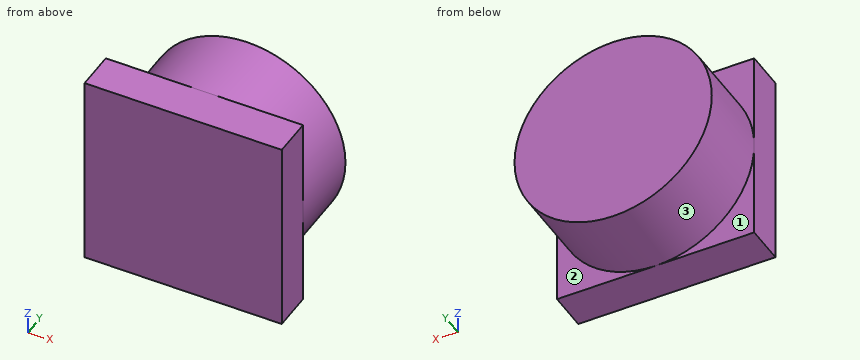
Autodesk Inventor part; units mm, degrees
ref_plane "YZ Plane" through (0, 0, 0) normal (1, 0, 0) x (0, 1, 0)
ref_plane "XZ Plane" through (0, 0, 0) normal (0, 1, 0) x (-1, 0, 0)
ref_plane "XY Plane" through (0, 0, 0) normal (0, 0, 1) x (1, 0, 0)
sketch "Skizze1" plane through (0, 0, 0) normal (0, 1, 0) x (-1, 0, 0)
  circle A0 centre (0, 0) radius 25
  dimension "d0" = 50
extrude "Extrusion1" add sketch "Skizze1" along normal blind 20
sketch "Skizze2" plane through (0, 0, 0) normal (0, -1, 0) x (1, 0, 0)
  line L0 (-25, 25) -> (25, 25)
  line L1 (25, 25) -> (25, -25)
  line L2 (25, -25) -> (-25, -25)
  line L3 (-25, -25) -> (-25, 25)
  circle A0 centre (0, 0) radius 25
extrude "Extrusion2" add sketch "Skizze2" along normal blind 10
equation "\"d0\" = UsedParameter"
equation "\"UsedParameter\" = 50"
equation "\"unusedParameter\" = 1"
properties part number "2Extrusionen"
Read the model definition and answer for the solid it produces. Units are mm, in the model's axes. Face numbers are marked on the shaded views. A direction names the side the tool comes from. Give positions to 0.01 mm unless a question says otherwise; leave off trailing zeros. Write each loop counter-clockwise with the first axis right and the second up, starting at its lowest first coordinate (ties: lowest second). Pieces come first, ordered by that corner, then holes. Notation, with made-up numbers: M 60,-25 L 82,-25 A33 cw 82,3 Z; hole C 42,4 d6. An arc over 180 degrees is marked long. Put each result on its own line as item: value. Start each with the question number.
1. The part is cut by section A-A, the plane x = 10.5. Give the vertices of the cut face in (y, z).
2. The part is cut by section B-B, the plane y = 8.25. Give the vertices of the cut face in (x, z).
3. Each of these flat-tipped pins is pushed along its axis until it touches: pin 1 Ø12 at (x, y) = (7.5, 8) entering from -Z; pin 2 Ø4 at (y, z) = (12.5, 6.5) entering from -X; pin 3 Ø10 at (y, z) = (14, -16) entering from +X. Where does it stop, or does it pass through?
4. Which of the six approach directions +Z, -Z, +X, -X, +Y, -Y give full straight-line access (tool end or side, diameter ignored) to the marked faces 1, 2 and 3?
5. Consider line 1 along Z through (x, y) = (-0.5, 8) (3 decimals); line 2 along Z through (x, y) = (-23, 0.5); line 3 along X through (y, z) = (6.75, -18.5). Determine where each line is inside the solid, lowest interval first.
Final values:
1. outline: M -10,-25 L 0,-25 L 0,-22.69 L 20,-22.69 L 20,22.69 L 0,22.69 L 0,25 L -10,25 Z
2. outline: C 0,0 d50
3. pin 1: stops at z = -24.95
3. pin 2: stops at x = -24.59
3. pin 3: stops at x = 22.45
4. face 1: -Z, -X, +Y
4. face 2: -Z, +X, +Y
4. face 3: +Y
5. line 1: z = -24.995 to 24.995
5. line 2: z = -9.8 to 9.8
5. line 3: x = -16.82 to 16.82
